Autodesk Inventor part; units mm, degrees
ref_plane "Work Plane1" through (0, 0, 41.275) normal (0, 0, -1) x (-1, 0, 0)
ref_plane "YZ Plane" through (0, 0, 0) normal (1, 0, 0) x (0, 1, 0)
ref_plane "XZ Plane" through (0, 0, 0) normal (0, 1, 0) x (-1, 0, 0)
sketch "Sketch1" plane through (0, 0, 0) normal (0, 0, 1) x (1, 0, 0)
  line L0 (2.2914, 3.9688) -> (4.5827, 0)
  line L1 (4.5827, 0) -> (2.2914, -3.9687)
  line L2 (2.2914, -3.9687) -> (-2.2914, -3.9687)
  line L3 (-2.2914, -3.9687) -> (-4.5827, 0)
  line L4 (-4.5827, 0) -> (-2.2914, 3.9688)
  line L5 (-2.2914, 3.9688) -> (2.2914, 3.9688)
  circle A0 centre (0, 0) radius 3.375
  dimension "d0" = 7.9375
  dimension "d1" = 6.75
extrude "Extrusion1" add sketch "Sketch1" along normal blind 101.6
sketch "Sketch2" plane through (0, 0, 0) normal (0, 0, -1) x (-1, 0, 0)
  circle A0 centre (0, 0) radius 3.925
  line L0 (2.2914, 3.9688) -> (4.5827, 0)
  line L1 (-2.2914, 3.9688) -> (2.2914, 3.9688)
  line L2 (-4.5827, 0) -> (-2.2914, 3.9688)
  line L3 (-2.2914, -3.9687) -> (-4.5827, 0)
  line L4 (2.2914, -3.9687) -> (-2.2914, -3.9687)
  line L5 (4.5827, 0) -> (2.2914, -3.9687)
  circle A1 centre (0, 0) radius 3.375
  dimension "d4" = 7.85
extrude "Extrusion2" cut sketch "Sketch2" against normal blind 25.4 contours L0 L5 L4 L3 L2 L1
ref_plane "Work Plane1" through (0, 0, 41.275) normal (0, 0, -1) x (-1, 0, 0)
sketch "Sketch3" plane through (0, 0, 41.275) normal (0, 0, -1) x (-1, 0, 0)
  line L0 (-4.5827, 0) -> (-2.2914, 3.9688)
  line L1 (-2.2914, -3.9687) -> (-4.5827, 0)
  line L2 (2.2914, -3.9687) -> (-2.2914, -3.9687)
  line L3 (4.5827, 0) -> (2.2914, -3.9687)
  line L4 (2.2914, 3.9688) -> (4.5827, 0)
  line L5 (-2.2914, 3.9688) -> (2.2914, 3.9688)
  circle A0 centre (0, 0) radius 3.925
  circle A1 centre (0, 0) radius 3.9688
  point P0 (-3.437, -1.9844)
  point P1 (-3.437, 1.9844)
  point P2 (0, 3.9688)
  point P3 (3.437, 1.9844)
  point P4 (3.437, -1.9844)
  point P5 (0, -3.9688)
extrude "Extrusion3" cut sketch "Sketch3" against normal through all contours L0 A1 L1 | L0 L5 A1 | A1 L2 L1 | L5 L4 A1 | A1 L3 L2 | L4 L3 A1
properties part number "Shaft" material "Stainless Steel"
For this review, take the finished solid that the model builds, in its own axes (mm). A direction names the side the tool comes from. Round coordinates to 2 decimals unless told otherwise and drop trailing zeros. Order: outer loops, then holes, each group sorted by start corner. A loop starts at its lowest first (then second) coordinate and runs counter-clockwise, first axis right, second up.
Q1. Wall thickness on line 1 (Y direction, x = 0, z = 37.5) (3 decimals); line 2 (X direction, y = 0.75, z = 45); line 3 (X direction, y = 3, z = 32.5): over which ranges is each line inside the solid? List them lowest first.
Findings below:
line 1: y = -3.969 to -3.375, 3.375 to 3.969
line 2: x = -3.9 to -3.29, 3.29 to 3.9
line 3: x = -2.85 to -1.55, 1.55 to 2.85
Q2. We need section A-A, the plane y = 1. Give the boundary of the cut face in (x, z) (3 decimals).
Findings below:
outline: (-4.005, 25.4) - (-3.795, 25.4) - (-3.795, 0) - (-3.223, 0) - (-3.223, 101.6) - (-3.841, 101.6) - (-3.841, 41.275) - (-4.005, 41.275) - close; (3.223, 0) - (3.795, 0) - (3.795, 25.4) - (4.005, 25.4) - (4.005, 41.275) - (3.841, 41.275) - (3.841, 101.6) - (3.223, 101.6) - close
Q3. We need section B-B, the plane x = 1.25. Give the boundary of the cut face in (y, z) (3 decimals), plus the area to 3 significant figures.
Findings below:
outline: (-3.969, 25.4) - (-3.721, 25.4) - (-3.721, 0) - (-3.135, 0) - (-3.135, 101.6) - (-3.767, 101.6) - (-3.767, 41.275) - (-3.969, 41.275) - close; (3.135, 0) - (3.721, 0) - (3.721, 25.4) - (3.969, 25.4) - (3.969, 41.275) - (3.767, 41.275) - (3.767, 101.6) - (3.135, 101.6) - close
area: 132 mm2
Q4. Insertion check: P1, Ø1, axis at y = -1.5, z = 46.5, coming from the -X side; P2, Ø3, axis at y = -2, z = 70, coming from the -X side; P3, Ø0.9, axis at x = 4.5, y = 0.5, coming from the +Z side (3 decimals). Each pin has a flat end and moves straight along its axis. Give the tip position at first contact, or say it passes through.
Findings below:
P1: stops at x = -3.84
P2: stops at x = -3.94
P3: stops at z = 41.275
Q5. We need section C-C, the plane z = 14. Give the boundary of the cut face in (x, y) (3 decimals), plus the area to 3 significant figures.
Findings below:
outline: circle Ø7.85 at (0, 0); hole circle Ø6.75 at (0, 0)
area: 12.6 mm2
Q6. Machinability: for faces 1 (the flat face through (-4.1, 0, 25.4)), 2 (the flat face through (-2.1, 3.6, 41.275)), 3 (the flat face through (2.1, -3.6, 41.275)), 4 (the flat face through (-2.1, -3.6, 41.275)), which of the approach directions +Z, -Z, +X, -X, +Y, -Y give a long, thin tool a straight path to every point of the face, cutting with its end or side? Answer none if there is none.
Findings below:
face 1: -Z
face 2: +Z, -X, +Y
face 3: +Z, +X, -Y
face 4: +Z, -X, -Y
Q7. Mouldability with a two-part tool opening along X and no side actions: class faces 5 (the flat face through (-3.42, -2.01, 33.23)), 6 (the cylindrical face through (2.893, 2.653, 12.522)), 7 (the flat face through (0, -3.969, 33)), 8 (the cylindrical face through (-0.7, 3.3, 50.1)) as pulls with the +X half, pulls with the -X half, needs draft (parallel to the pull), parting line crosses it, or undercut.
Findings below:
face 5: pulls with the -X half
face 6: parting line crosses it
face 7: needs draft
face 8: undercut
Q8. We need section D-D, the plane z = 44.5. Give the boundary of the cut face in (x, y) (3 decimals).
Findings below:
outline: circle Ø7.938 at (0, 0); hole circle Ø6.75 at (0, 0)
